The figure shows three views and two pictorial views of one solid part (mm, origin at its lowest corner). Answer the questions. Coordinates: 2 decimals unless noted, no trailing zeros. Write each loop counter-clockwise with the first axis right and the second up, starting at its lowest first coordinate (ties: lowest second). Pieces come first, ordered by that corner, then holes.
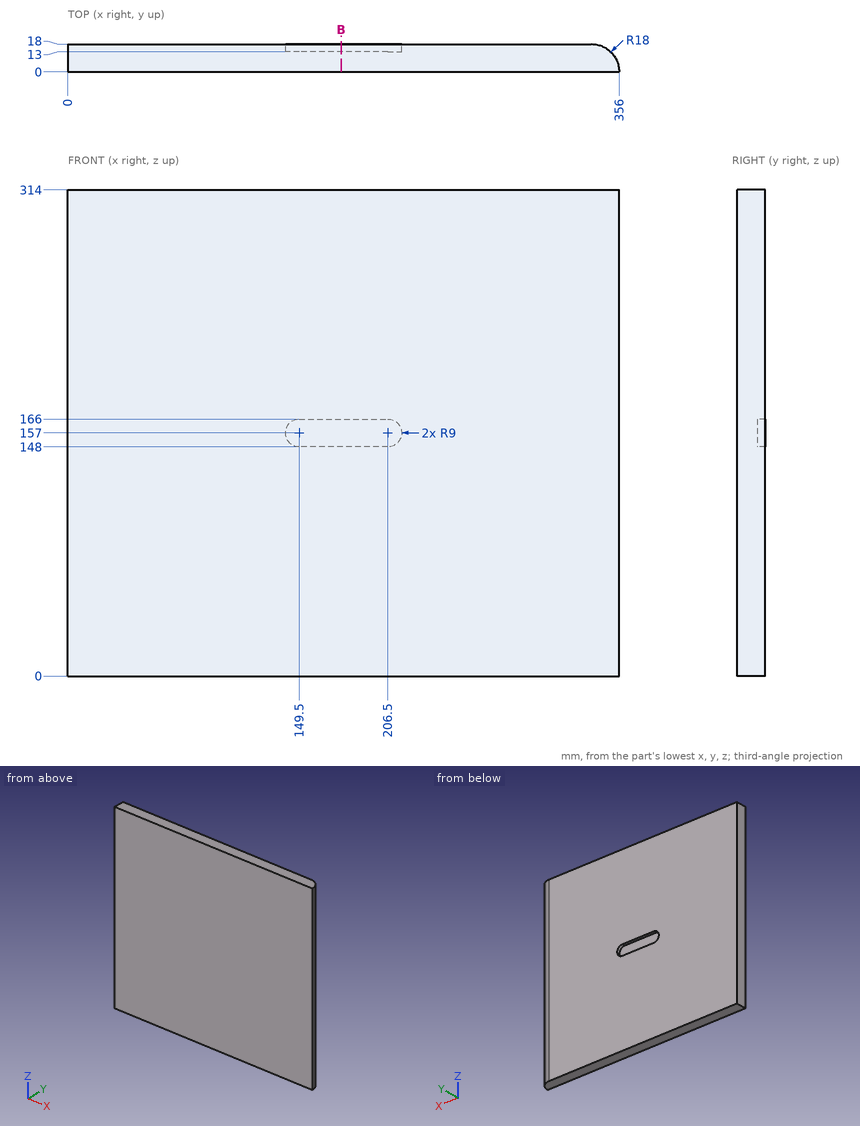
1. Find the intervals of material crossed by L1, parallel to Z at x = 184.5, y = 15; L2, parallel to X at y = 1.5, z = 156; L3, parallel to X at y = 1, z = 73, in increasing order.
Results found:
L1: z = 0 to 148, 166 to 314
L2: x = 0 to 355.94
L3: x = 0 to 355.97
2. A flat-ended cylindrical pin translates along its axis: P1, Ø4, axis at y = 15, z = 277.5, coming from the +X side. Find the tip coordinate at first contact, or state that the pin passes through.
Results found:
P1: stops at x = 350.45
3. Section B-B on x = 176.5 is taken. Give the vertices of the cut face in (y, z).
Results found:
outline: (0, 0) - (18, 0) - (18, 148) - (13, 148) - (13, 166) - (18, 166) - (18, 314) - (0, 314) - close
